Source: CAD feature listing. Evaluate the final solid. Frame: model axes, mm. A direction names the side the tool comes from. Round coordinates to 2 decimals unless told otherwise and drop trailing zeros. Write each loop counter-clockwise with the first axis right and the second up, starting at its lowest first coordinate (ties: lowest second). Pieces come first, ordered by that corner, then holes. Notation, with made-up numbers: M 10.5,55 L 58.5,55 A16 cw 58.5,75 Z; hole C -28.75,23 d8. An arc over 180 degrees is marked long. Answer in a Markdown table with one row per item. Add a question column.
Item 1: Cut plane B-B on y = 0. Return loops of the section in (x, z).
Item 2: Set-up query: faces 4 (the face through (-2.03, -3.04, -3.32)), 5 (the face through (0, 0, 0)), 6 (the face through (-14, -4, 15)), 7 (the face through (-6.5, -0.1, -2.5)). Return all of +Z, -Z, +X, -X, +Y, -Y with unobstructed straight access to the full face (end or side cutting, diameter ignored); none if empty.
Item 3: Cut plane C-C on x = -5.5. Return loops of the section in (y, z).
Item 4: Mould query, pull axis Y, two halves, no side actions, for faces 1 (the face through (-14, 0, 26)), 2 (the face through (-10, 3, -3)), 3 (the face through (-19, 0, 0)). Classes: released by +Y, released by -Y, zero draft, split by the parting line, or undercut.
Item 5: Cut plane A-A on z = 0. Return loops of the section in (x, y).
Item 6: Contact query for flat-ended pins moving along their axis: pin 1 (4.5 mm diameter, centred on x = -24.25, z = 0, fed in from -Y); pin 2 (3 mm diameter, centred on x = -23, z = -1.5, fed in from +Y); pin 3 (0.9 mm diameter, centred on x = -13.5, z = 17, fed in from +Y); pin 4 (1.4 mm diameter, centred on y = 0, z = 2.5, fed in from -X). Output: stop coordinate, or through.
Item 7: Material intervals for probe 1 along X at (y, z) = (-4.3, 0); probe 2 along X at (y, z) = (-2.75, 3); probe 3 along X at (y, z) = (0.25, 22.5), sorted ascending.
from build123d import *

# Parameters (mm, degrees)
SKETCH2_W               = 20.869986484
SKETCH2_H               = 4.5
CUT_EXTRUDE1_DEPTH      = 12
CUT_EXTRUDE2_DEPTH      = 33.14031736
CUT_EXTRUDE2_DEPTH_BACK = 33.14031736
SKETCH3_R               = 2.75
BOSS_EXTRUDE1_START     = -15
BOSS_EXTRUDE1_DEPTH     = 3
SKETCH6_R               = 2.5
BOSS_EXTRUDE2_DEPTH     = 22
FILLET1_R               = 1
FILLET2_R               = 1.5


# Read off the part's stored shape, not the designer's step: Boss-Extrude1
with BuildPart() as part:
    # Sketch1 → Revolve1 (revolve)
    with BuildSketch(Plane(origin=(0, 0, 0), x_dir=(1, 0, 0), z_dir=(0, 1, 0)), mode=Mode.PRIVATE) as revolve1_sk:
        Polygon((0, 0), (0, 4.5), (-4, 4.5), (-4, 2.5), (-10, 2.5), (-10, 6), (-31, 6), (-31, 0), align=None)
    revolve(revolve1_sk.sketch.rotate(Axis((-13.308467742, 0, 0), (1, 0, 0)), 180), axis=Axis((-13.308467742, 0, 0), (1, 0, 0)))

    # Sketch2 → Cut-Extrude1 (cut)
    with BuildSketch(Plane.ZY.offset(31)):
        Rectangle(SKETCH2_W, SKETCH2_H)
    extrude(amount=-CUT_EXTRUDE1_DEPTH, mode=Mode.SUBTRACT)

    # Sketch3 → Cut-Extrude2 (cut, two sides: drawn at the far end of the back side and taken through both)
    with BuildSketch(Plane(origin=(0, 0, 0), x_dir=(1, 0, 0), z_dir=(0, 1, 0)).offset(-CUT_EXTRUDE2_DEPTH_BACK)):
        with Locations(Location((-24.25, 0, 0), (0, 0, 270))):
            Circle(SKETCH3_R)
    extrude(amount=CUT_EXTRUDE2_DEPTH + CUT_EXTRUDE2_DEPTH_BACK, mode=Mode.SUBTRACT)

    # Boss-Extrude1 outline → Boss-Extrude1 (add)
    with BuildSketch(Plane.YZ.offset(BOSS_EXTRUDE1_START)):
        with BuildLine():
            ThreePointArc((4, 24.472135955), (0, 26), (-4, 24.472135955))
            Line((-4, 24.472135955), (-4, 4.472135955))
            ThreePointArc((-4, 4.472135955), (0, 6), (4, 4.472135955))
            Line((4, 4.472135955), (4, 24.472135955))
        make_face()
    extrude(amount=BOSS_EXTRUDE1_DEPTH)

    # Sketch6 → Boss-Extrude2 (add)
    with BuildSketch(Plane(origin=(-12, 0, 0), x_dir=(0, 0, -1), z_dir=(1, 0, 0))):
        with Locations((-21.5, 0)):
            Circle(SKETCH6_R)
    extrude(amount=BOSS_EXTRUDE2_DEPTH)

    # Fillet1
    fillet1_edges = [part.edges().sort_by_distance(p)[0] for p in [
        (-10, 0, -2.5),
    ]]
    fillet(fillet1_edges, radius=FILLET1_R)

    # Fillet2
    fillet2_edges = [part.edges().sort_by_distance(p)[0] for p in [
        (-12, 0, 24),
    ]]
    fillet(fillet2_edges, radius=FILLET2_R - 0.0001)  # a hair under: the kernel refuses the full size


solid = part.part
Results below:
| question | item | result |
|---|---|---|
| 1 | outline | M -19,-6 L -10,-6 L -10,-3.5 A1 cw -9,-2.5 L -4,-2.5 L -4,-4.5 L 0,-4.5 L 0,4.5 L -4,4.5 L -4,2.5 L -9,2.5 A1 cw -10,3.5 L -10,6 L -12,6 L -12,17.5 A1.5 cw -10.5,19 L 10,19 L 10,24 L -10.5,24 A1.5 cw -12,25.5 L -12,26 L -15,26 L -15,6 L -19,6 Z |
| 2 | face 4 | +X |
| 2 | face 5 | -Z, +X, +Y, -Y |
| 2 | face 6 | +Z, +X, -X, -Y |
| 2 | face 7 | none |
| 3 | outline | C 0,0 d5; C 0,21.5 d5 |
| 4 | face 1 | split by the parting line |
| 4 | face 2 | zero draft |
| 4 | face 3 | undercut |
| 5 | outline | M -31,-6 L -27,-6 L -27,-2.25 L -31,-2.25 Z; M -31,2.25 L -27,2.25 L -27,6 L -31,6 Z; M -21.5,-6 L -10,-6 L -10,-3.5 A1 cw -9,-2.5 L -4,-2.5 L -4,-4.5 L 0,-4.5 L 0,4.5 L -4,4.5 L -4,2.5 L -9,2.5 A1 cw -10,3.5 L -10,6 L -21.5,6 L -21.5,2.25 L -19,2.25 L -19,-2.25 L -21.5,-2.25 Z |
| 6 | pin 1 | through |
| 6 | pin 2 | y = 5.94 |
| 6 | pin 3 | y = 4 |
| 6 | pin 4 | x = -19 |
| 7 | probe 1 | -31 to -27, -21.5 to -10, -4 to 0 |
| 7 | probe 2 | -31 to -10, -4 to 0 |
| 7 | probe 3 | -15 to 10 |
